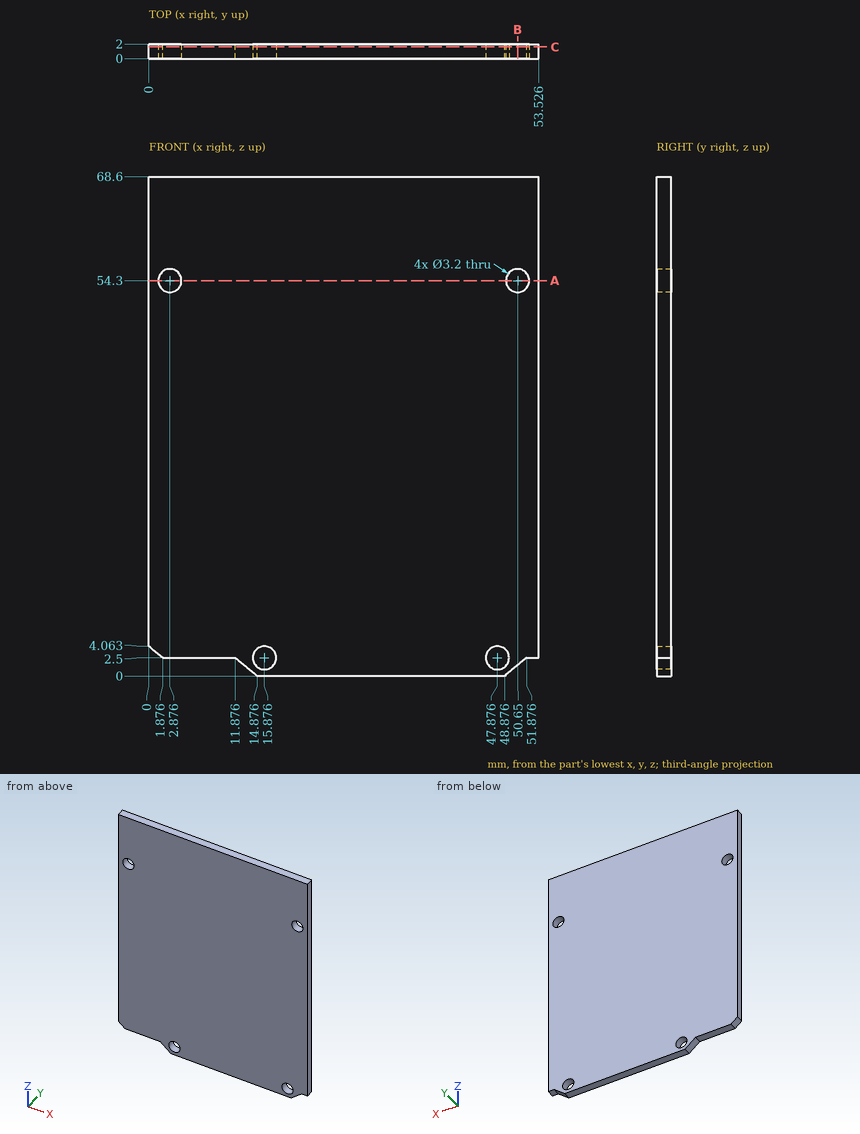
For this review, use the dimensioned drawing (mm, ordinates from the lowest corner) and the shaded views. Give positions to 0.01 mm unless a question says otherwise; leave off trailing zeros. Loops run counter-clockwise (first coordinate to the right, second up) from the corner with the lowest first, then second, coordinate; pieces in that order, holes last. Notation, with made-up numbers: (-22.5, 1) - (18.5, 1) arc R15 ccw to (18.5, 7) - close; hole circle Ø7 at (27.5, 82.25). An arc over 180 degrees is marked (long way). Write each question's results on one line, items separated by ' | '.
(1) For line 1 along X through (y, z) = (0.6, 54.3); line 2 along Z through (x, y) = (48, 1) (1 decimal); line 3 along Z through (x, y) = (51, 0.5), list the stretches that pass through material, from the lowest coordinate up.
Conclusion:
line 1: 0 to 1.28, 4.48 to 49.05, 52.25 to 53.53 | line 2: 0 to 0.9, 4.1 to 68.6 | line 3: 1.77 to 52.74, 55.86 to 68.6
(2) Take a section at B-B (x = 50.65). Give the boundary of the cut face in (y, z), then the cut area to 3 significant figures.
Conclusion:
outline: (0, 1.48) - (2, 1.48) - (2, 52.7) - (0, 52.7) - close; (0, 55.9) - (2, 55.9) - (2, 68.6) - (0, 68.6) - close | area: 128 mm^2
(3) For pin 1 Ø1.9 at (x, z) = (2.88, 54.3) entering from +Y; pin 2 Ø1 at (x, y) = (7, 0.5) entering from -Z; pin 3 Ø8 at (x, z) = (27.5, 22.5) entering from -Y, all flat-tipped, find the tip position at first contact; note any pin that passes through.
Conclusion:
pin 1: through | pin 2: z = 2.5 | pin 3: y = 0
(4) Take a section at C-C (y = 1.6). Give the boundary of the cut face in (x, z).
Conclusion:
outline: (0, 4.06) - (1.88, 2.5) - (11.88, 2.5) - (14.88, 0) - (48.88, 0) - (51.88, 2.5) - (53.53, 2.5) - (53.53, 68.6) - (0, 68.6) - close; hole circle Ø3.2 at (2.88, 54.3); hole circle Ø3.2 at (15.88, 2.5); hole circle Ø3.2 at (47.88, 2.5); hole circle Ø3.2 at (50.65, 54.3)
(5) Take a section at A-A (z = 54.3). Give the boundary of the cut face in (x, y).
Conclusion:
outline: (0, 0) - (1.28, 0) - (1.28, 2) - (0, 2) - close; (4.48, 0) - (49.05, 0) - (49.05, 2) - (4.48, 2) - close; (52.25, 0) - (53.53, 0) - (53.53, 2) - (52.25, 2) - close
